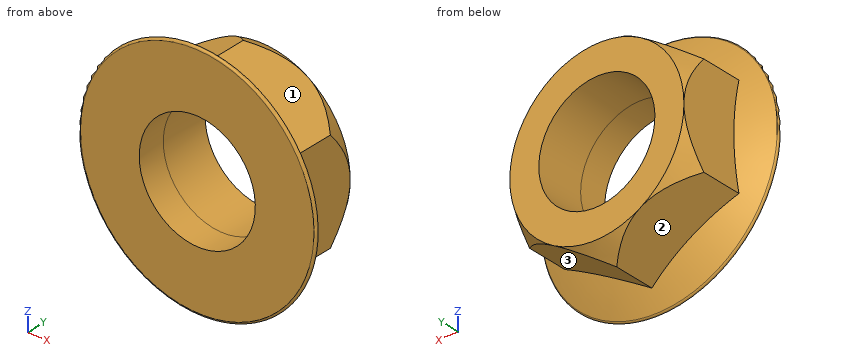
from build123d import *

# Parameters (mm, degrees)
SKETCH1_R           = 15
BOSS_EXTRUDE1_DEPTH = 20
SKETCH2_OUTSIDE_W   = 104.228
SKETCH2_OUTSIDE_H   = 104.228
SKETCH2_OUTSIDE_R   = 22.5
CUT_EXTRUDE1_DEPTH  = 20
CUT_EXTRUDE1_DRAFT  = -30
CUT_EXTRUDE2_REACH  = 49.758
SKETCH4_R           = 15


with BuildPart() as part:
    # Sketch1 → Boss-Extrude1 (new body)
    with BuildSketch(Plane(origin=(0, 0, 0), x_dir=(1, 0, 0), z_dir=(0, 1, 0))):
        Polygon((0, 25.980762114), (-22.5, 12.990381057), (-22.5, -12.990381057), (0, -25.980762114), (22.5, -12.990381057), (22.5, 12.990381057), align=None)
        with Locations(Location((0, 0, 0), (0, 0, 270))):
            Circle(SKETCH1_R, mode=Mode.SUBTRACT)
    extrude(amount=BOSS_EXTRUDE1_DEPTH)

    # Sketch3 → Revolve1 (revolve)
    with BuildSketch(Plane.XY, mode=Mode.PRIVATE) as revolve1_sk:
        with BuildLine():
            Line((0, 9.214199819), (0, 0))
            Line((0, 0), (30.166483054, 0))
            ThreePointArc((30.166483054, 0), (30.648917793, 0.368635156), (30.419982911, 0.930973111))
            ThreePointArc((30.419982911, 0.930973111), (15.763781312, 7.106368536), (0, 9.214199819))
        make_face()
    revolve(revolve1_sk.sketch.rotate(Axis((0, 0, 0), (0, -1, 0)), 90), axis=Axis((0, 0, 0), (0, -1, 0)))


with BuildPart() as cut_extrude1_tool:
    # Sketch2 outside → Cut-Extrude1 (with draft: the straight prism first)
    with BuildSketch(Plane(origin=(0, 20, 0), x_dir=(1, 0, 0), z_dir=(0, 1, 0))):
        Rectangle(SKETCH2_OUTSIDE_W, SKETCH2_OUTSIDE_H)
        Circle(SKETCH2_OUTSIDE_R, mode=Mode.SUBTRACT)
    extrude(amount=-CUT_EXTRUDE1_DEPTH)
    # Cut-Extrude1: the draft: its side faces are tilted about the plane it starts from
    cut_extrude1_sides = [cut_extrude1_tool.faces().sort_by_distance(p)[0] for p in [
        (0, 10, 52.114),
        (52.114, 10, 0),
        (0, 10, -52.114),
        (-52.114, 10, 0),
        (-22.5, 10, 0),
    ]]
    draft(cut_extrude1_sides, Plane(origin=(0, 20, 0), x_dir=(1, 0, 0), z_dir=(0, 1, 0)), CUT_EXTRUDE1_DRAFT)


with BuildPart() as part_1:
    add(part.part)

    # Cut-Extrude1: cut by cut_extrude1_tool
    add(cut_extrude1_tool.part, mode=Mode.SUBTRACT)

    # Sketch4 → Cut-Extrude2 (cut, up to next)
    with BuildSketch(Plane(origin=(0, 20, 0), x_dir=(1, 0, 0), z_dir=(0, 1, 0)), mode=Mode.PRIVATE) as cut_extrude2_sk1:
        with Locations(Location((0, 0, 0), (0, 0, 270))):
            Circle(SKETCH4_R)
    cut_extrude2_tool1 = extrude(cut_extrude2_sk1.sketch, amount=-CUT_EXTRUDE2_REACH, mode=Mode.PRIVATE) & part_1.part
    add(cut_extrude2_tool1.solids().sort_by_distance((0, 20, 0))[0], mode=Mode.SUBTRACT)


solid = part_1.part
Geometry: final body of the model. Coordinates: model frame, mm. Face numbers are marked on the shaded views. A direction names the side the tool comes from. Give positions to 0.01 mm unless a question says otherwise; leave off trailing zeros. Write each loop counter-clockwise with the first axis right and the second up, starting at its lowest first coordinate (ties: lowest second). Pieces come first, ordered by that corner, then holes. Notation, with made-up numbers: (69.5, 27) -> (124.5, 27) arc R32 ccw to (124.5, 62) -> close; hole circle Ø10 at (72, 51). An arc over 180 degrees is marked (long way). Answer as a JSON object with one key per item and string values.
1. Access query for the marked faces 1, 2 and 3. Directions: +Z, -Z, +X, -X, +Y, -Y. A direction counts if a zero-diameter tool reaches every point of the face in a straight line with its end or side. Return the directions, or none.
Ans:
{"face 1": "+Z, +X, +Y", "face 2": "-Z, -X, +Y", "face 3": "-Z, +X, +Y"}
2. Cut plane B-B on y = 17.75. Output: boundary loops of the cut face in (x, z), and give its area (3 significant figures).
Ans:
{"outline": "(-22.5, -7.76) arc R23.8 ccw to (-17.97, -15.61) -> (-4.53, -23.36) arc R23.8 ccw to (4.53, -23.36) -> (17.97, -15.61) arc R23.8 ccw to (22.5, -7.76) -> (22.5, 7.76) arc R23.8 ccw to (17.97, 15.61) -> (4.53, 23.36) arc R23.8 ccw to (-4.53, 23.36) -> (-17.97, 15.61) arc R23.8 ccw to (-22.5, 7.76) -> close; hole circle Ø30 at (0, 0)", "area": "991 mm^2"}
3. Ray query, probe 1 along Z at (x, y) = (0, 4.25); probe 2 along X at (y, z) = (11.75, 11.5); probe 3 along Z at (x, y) = (2, 10). Return the intervals inside material, ascending. Write a range as from..to.
Ans:
{"probe 1": "z = -25.98..-15, 15..25.98", "probe 2": "x = -22.5..-9.63, 9.63..22.5", "probe 3": "z = -24.83..-14.87, 14.87..24.83"}
4. Contact query for flat-ended pins moving along their axis: pin 1 (6 mm diameter, centred on x = 9.5, z = -13.5, fed in from -Y); pin 2 (2 mm diameter, centred on y = 9, z = -20.5, fed in from -X) (3 decimals); pin 3 (10 mm diameter, centred on y = 13.5, z = -11, fed in from -X); pin 4 (4 mm diameter, centred on y = 13.5, z = 22, fed in from -X). Output: stop coordinate, or through.
Ans:
{"pin 1": "stops at y = 0", "pin 2": "stops at x = -11.225", "pin 3": "stops at x = -22.5", "pin 4": "stops at x = -10.36"}
5. Cut plane A-A on y = 8.25. Output: boundary loops of the cut face in (x, z).
Ans:
{"outline": "(-22.5, -12.99) -> (0, -25.98) -> (22.5, -12.99) -> (22.5, 12.99) -> (0, 25.98) -> (-22.5, 12.99) -> close; hole circle Ø30 at (0, 0)"}
